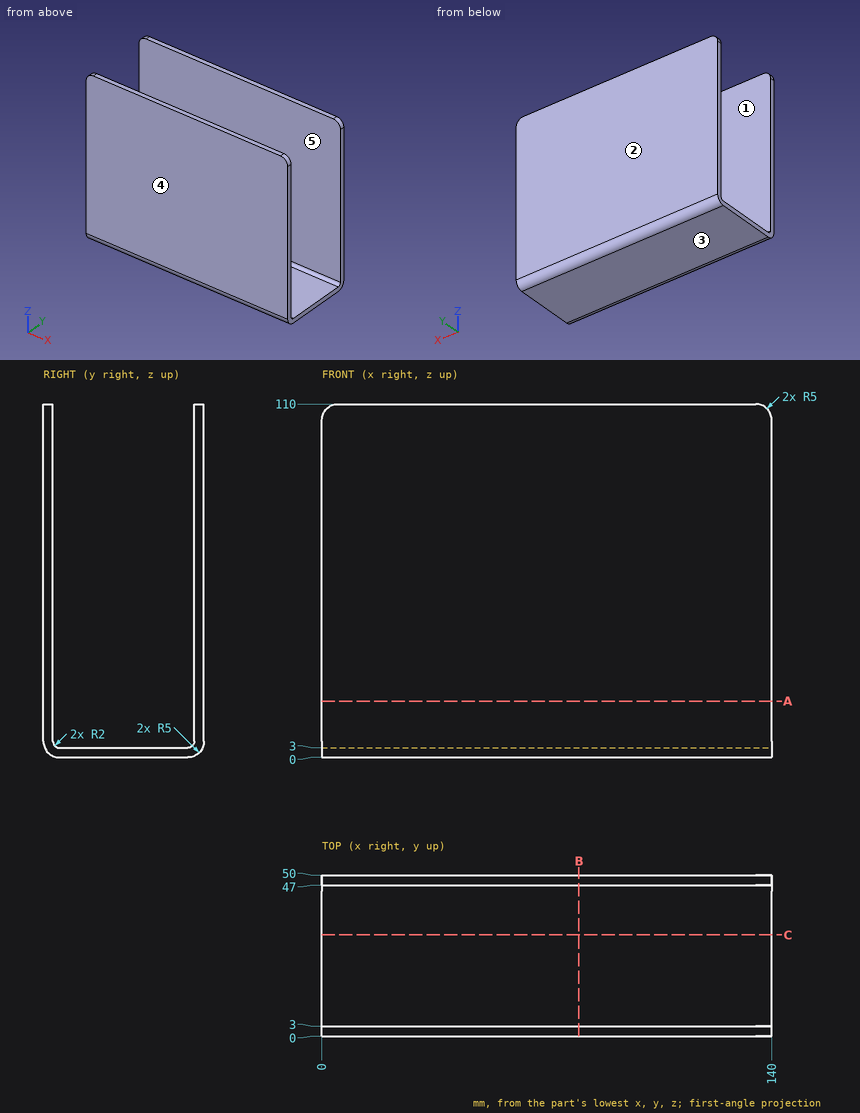
Can you work these out from the drawing? Everything is in mm from the part's minimum corner. A direction names the side the tool comes from. Round coordinates to 2 decimals unless told otherwise and drop trailing zeros. Write each loop counter-clockwise with the first axis right and the second up, starting at its lowest first coordinate (ties: lowest second). Pieces come first, ordered by that corner, then holes. Notation, with made-up numbers: (-21, 9.25) - (38, 9.25) arc R26 ccw to (38, 31.25) - close; hole circle Ø11 at (58, -25.75). An arc over 180 degrees is marked (long way). Use a Markdown table: item, result.
Q1. Please list where these lines run through material, in increasing order: L1, parallel to Y at x = 130, z = 47; L2, parallel to Z at x = 105.5, y = 21.5.
Output values:
| item | result |
|---|---|
| L1 | 0 to 3, 47 to 50 |
| L2 | 0 to 3 |
Q2. I want a section at A-A (z = 17.5). List the corners of the cut face in (x, y) for me, plus the area to 3 significant figures.
Output values:
| item | result |
|---|---|
| outline | (0, 0) - (140, 0) - (140, 3) - (0, 3) - close; (0, 47) - (140, 47) - (140, 50) - (0, 50) - close |
| area | 840 mm2 |
Q3. Thinking about a two-plate mould opening in Y: for the marked faces 1, 2 and 3, which applies, released by +Y, released by -Y, zero draft, split by the parting line, or undercut?
Output values:
| item | result |
|---|---|
| face 1 | undercut |
| face 2 | released by +Y |
| face 3 | zero draft |
Q4. For pin 1 (12 mm diameter, centred on x = 53, y = 16.5, fed in from +Z), with a flat end and sliding along its axis, tell me the tip position at first contact or that it passes through.
Output values:
| item | result |
|---|---|
| pin 1 | z = 3 |
Q5. I want a section at B-B (x = 80). List the corners of the cut face in (y, z) for me, plus the area to 3 significant figures.
Output values:
| item | result |
|---|---|
| outline | (0, 5) arc R5 ccw to (5, 0) - (45, 0) arc R5 ccw to (50, 5) - (50, 110) - (47, 110) - (47, 5) arc R2 cw to (45, 3) - (5, 3) arc R2 cw to (3, 5) - (3, 110) - (0, 110) - close |
| area | 783 mm2 |
Q6. For the marked faces 4 and 5, which set-ups out of +Z, -Z, +X, -X, +Y, -Y let a thin tool reach every point of the face, with its end or its side?
Output values:
| item | result |
|---|---|
| face 4 | +Z, -Z, +X, -X, -Y |
| face 5 | +Z, +X, -X |
Q7. I want a section at C-C (y = 31.5). List the corners of the cut face in (x, z) for me.
Output values:
| item | result |
|---|---|
| outline | (0, 0) - (140, 0) - (140, 3) - (0, 3) - close |
